```python
from build123d import *

# Parameters (mm, degrees)
SKETCH003_R     = 1.75
SKETCH004_R     = 4
PAD_DEPTH       = 3
SKETCH001_R     = 3.1
POCKET_DEPTH    = 2.3
SKETCH002_R     = 2
POCKET001_DEPTH = 3.001


with BuildPart() as obj1:
    # Sketch003 → Loft section 0
    with BuildSketch(Plane.YZ.offset(0.5)):
        with Locations((0, 10.05)):
            Circle(SKETCH003_R)
    # Sketch004 → Loft section 1
    with BuildSketch(Plane.YZ.offset(3.5)):
        with Locations((0, 10.05)):
            Circle(SKETCH004_R)
    loft()


with BuildPart() as cut:
    # Sketch → Pad (new body)
    with BuildSketch(Plane.YZ):
        with BuildLine():
            Line((-5.993983, 9.781369), (-5.544434, -0.248507))
            ThreePointArc((-5.544434, -0.248507), (0, -5.55), (5.544434, -0.248507))
            Line((5.993983, 9.781369), (5.544434, -0.248507))
            ThreePointArc((5.993983, 9.781369), (0, 16.05), (-5.993983, 9.781369))
        make_face()
    extrude(amount=PAD_DEPTH)

    # Sketch001 → Pocket (cut)
    with BuildSketch(Plane(origin=(0, 0, 0), x_dir=(0, 1, 0), z_dir=(-1, 0, 0))):
        Circle(SKETCH001_R)
    extrude(amount=-POCKET_DEPTH, mode=Mode.SUBTRACT)

    # Sketch002 → Pocket001 (cut, through all)
    with BuildSketch(Plane.YZ.offset(3)):
        with Locations((0, 10.05)):
            Circle(SKETCH002_R)
    extrude(amount=-POCKET001_DEPTH, mode=Mode.SUBTRACT)

    # Cut: cut obj1
    add(obj1.part, mode=Mode.SUBTRACT)


solid = cut.part
```
Could you check a few things on this model? Use its own coordinates, in mm. A direction names the side the tool comes from. Give positions to 0.01 mm unless a question says otherwise; leave off trailing zeros. Order: outer loops, then holes, each group sorted by start corner. A loop starts at its lowest first (then second) coordinate and runs counter-clockwise, first axis right, second up.
Q1. For faces 1 (the cylindrical face through (1.13, 1.43, 2.75)), 2 (the flat face through (1.479, -5.772, 4.837)), which set-ups out of +Z, -Z, +X, -X, +Y, -Y let a thin tool reach every point of the face, with its end or its side?
Q2. We'd pull the mould along Z, two halves only. Please class faces 3 (the flat face through (1.479, 5.772, 4.837)), 4 (the flat face through (2.3, 0, 0)), 5 (the flat face through (3, 0, 5)), 6 (the conical face through (0.97, -2.1, 10.14)): +Z half, -Z half, draft (parallel to the pull), parting line (faces both ways), or undercut.
Q3. I'm going to push flat-ended pins straight in: P1, Ø1.5, axis at y = 1, z = 10, coming from the -X side; P2, Ø6.5, axis at y = 0, z = 10.05, coming from the -X side; P3, Ø3, axis at y = 1.5, z = 9.5, coming from the +X side; P4, Ø4, axis at y = -1, z = 11, coming from the +X side. Where does each tip first touch, or does it pass through?
Q4. Suppose I cut it at C-C, the plane z = 0. Write out the boundary of the cut face in (x, y).
Q5. Suppose I cut it at B-B, the plane x = 0.5. Write out the boundary of the cut face in (y, z), and give its area (3 significant figures).
Q6. Suppose I cut it at A-A, the plane y = 0. Write out the boundary of the cut face in (x, z) (3 decimals), and give its area (3 significant figures).
Q7. If I drill on line 1 along Z through (x, y) = (1.95, 2); line 2 along Y through (x, z) = (0.5, 10.05); line 3 along Y through (x, z) = (0.5, 10.5), over which ranges is the centre line in solid material (lowest first)?
Solution:
1. face 1: -X
1. face 2: -Z, +X, -X, -Y
2. face 3: -Z half
2. face 4: undercut
2. face 5: draft
2. face 6: undercut
3. P1: passes through
3. P2: stops at x = 0
3. P3: stops at x = 2.3
3. P4: stops at x = 2.67
4. outline: (0, -5.56) - (3, -5.56) - (3, 5.56) - (0, 5.56) - (0, 3.1) - (2.3, 3.1) - (2.3, -3.1) - (0, -3.1) - close
5. outline: (-5.99, 9.78) - (-5.54, -0.25) arc R5.55 ccw to (5.54, -0.25) - (5.99, 9.78) arc R6 ccw (long way) to start; hole circle Ø6.2 at (0, 0); hole circle Ø4 at (0, 10.05)
5. area: 178 mm2
6. outline: (0, -5.55) - (3, -5.55) - (3, 6.425) - (0.833, 8.05) - (0, 8.05) - (0, 3.1) - (2.3, 3.1) - (2.3, -3.1) - (0, -3.1) - close; (0, 12.05) - (0.833, 12.05) - (3, 13.675) - (3, 16.05) - (0, 16.05) - close
6. area: 35.0 mm2
7. line 1: z = -5.18 to -2.37, 2.37 to 8.04, 12.06 to 15.71
7. line 2: y = -6 to -2, 2 to 6
7. line 3: y = -5.98 to -1.95, 1.95 to 5.98
